CAD build for the part. Positions are in the model's coordinates, mm. Give positions to 0.01 mm unless a question says otherwise; leave off trailing zeros. Loops run counter-clockwise (first coordinate to the right, second up) from the corner with the lowest first, then second, coordinate; pieces in that order, holes last.
Item 1: Saw through at B-B on y = 0.45. Give the cut face in (x, z).
Item 2: Probe probe 1 along X at (y, z) = (1.3, 92.5); probe 2 along Z at (x, y) = (-97, 0.9); probe 3 along X at (y, z) = (0.25, 11). List the from-to ranges inside material, lowest first.
Item 3: Saw through at C-C on z = 49.5. Give the cut face in (x, y).
Item 4: Drop flat-ended pins along their axis: P1, Ø0.9, axis at y = 1.5, z = -33.5, coming from the -X side; P2, Ø1, axis at y = 1.5, z = -2.5, coming from the +X side. Give the stop position or say it passes through.
Item 5: Saw through at A-A on x = 95. Give the cut face in (y, z), plus the area to 3 significant figures.
from build123d import *

# Parameters (mm, degrees)
SKETCH1_W           = 272
SKETCH1_H           = 220
BOSS_EXTRUDE1_DEPTH = 3
SKETCH2_OUTSIDE_W   = 343.97
SKETCH2_OUTSIDE_H   = 291.97
CUT_EXTRUDE1_DEPTH  = 175.94284781
SKETCH3_R           = 1.5
CUT_EXTRUDE2_DEPTH  = 175.94284781
SKETCH5_R           = 1.5
CUT_EXTRUDE4_DEPTH  = 175.94284781


with BuildPart() as part:
    # Sketch1 → Boss-Extrude1 (new body)
    with BuildSketch(Plane(origin=(0, 0, 0), x_dir=(1, 0, 0), z_dir=(0, 1, 0))):
        Rectangle(SKETCH1_W, SKETCH1_H)
    extrude(amount=BOSS_EXTRUDE1_DEPTH)

    # Sketch2 outside → Cut-Extrude1 (cut, through all)
    with BuildSketch(Plane(origin=(0, 3, 0), x_dir=(1, 0, 0), z_dir=(0, 1, 0))):
        Rectangle(SKETCH2_OUTSIDE_W, SKETCH2_OUTSIDE_H)
        Polygon((-136, 110), (136, 110), (136, 75), (35, 75), (35, -75), (136, -75), (136, -110), (-136, -110), (-136, -75), (-35, -75), (-35, 75), (-136, 75), align=None, mode=Mode.SUBTRACT)
    extrude(amount=-CUT_EXTRUDE1_DEPTH, mode=Mode.SUBTRACT)

    # Sketch3 → Cut-Extrude2 (cut, through all)
    with BuildSketch(Plane.XZ):
        with Locations(Location((25, 92.5, 0), (0, 0, 270))):
            Circle(SKETCH3_R)
        with Locations(Location((-25, 92.5, 0), (0, 0, 270))):
            Circle(SKETCH3_R)
    extrude(amount=-CUT_EXTRUDE2_DEPTH, mode=Mode.SUBTRACT)

    # Sketch5 → Cut-Extrude4 (cut, through all)
    with BuildSketch(Plane.XZ):
        with Locations(Location((0, 88.5, 0), (0, 0, 270))):
            Circle(SKETCH5_R)
    extrude(amount=-CUT_EXTRUDE4_DEPTH, mode=Mode.SUBTRACT)


solid = part.part
Results below:
1. outline: (-136, -110) - (136, -110) - (136, -75) - (35, -75) - (35, 75) - (136, 75) - (136, 110) - (-136, 110) - (-136, 75) - (-35, 75) - (-35, -75) - (-136, -75) - close; hole circle Ø3 at (-25, 92.5); hole circle Ø3 at (0, 88.5); hole circle Ø3 at (25, 92.5)
2. probe 1: x = -136 to -26.5, -23.5 to 23.5, 26.5 to 136
2. probe 2: z = -110 to -75, 75 to 110
2. probe 3: x = -35 to 35
3. outline: (-35, 0) - (35, 0) - (35, 3) - (-35, 3) - close
4. P1: stops at x = -35
4. P2: stops at x = 35
5. outline: (0, -110) - (3, -110) - (3, -75) - (0, -75) - close; (0, 75) - (3, 75) - (3, 110) - (0, 110) - close
5. area: 210 mm2
